Here's the drawing with two shaded views (mm, measured from the low corner). I have some questions. Give positions to 0.01 mm unless a question says otherwise; leave off trailing zeros. Loops run counter-clockwise (first coordinate to the right, second up) from the corner with the lowest first, then second, coordinate; pieces in that order, holes last. Notation, with made-up numbers: (-29, 23.25) -> (11, 23.25) arc R32 ccw to (11, 52.25) -> close; hole circle Ø6 at (40, 81). An arc over 180 degrees is marked (long way). Answer in a Markdown table with one row per item. Add a question column.
Item 1: If we section it at D-D (x = 72): Write out the boundary of the cut face in (y, z).
Item 2: For P1, Ø1.5, axis at y = 1, z = 13.5, coming from the +X side (1 decimal); P2, Ø3, axis at x = 73, y = 1.5, coming from the -Z side, each with a flat end and sliding along its axis, tell me the tip position at first contact or that it passes through.
Item 3: If we section it at C-C (z = 19): Write out the boundary of the cut face in (x, y), then the cut area to 3 significant figures.
Item 4: If we section it at B-B (z = 35.5): Write out the boundary of the cut face in (x, y) (1 decimal).
Item 5: If we section it at A-A (y = 3.3): Write out the boundary of the cut face in (x, z) (1 decimal).
Item 6: If I drill on line 1 (Z direction, x = 47.5, y = 4.45) (1 decimal); line 2 (Z direction, x = 44, y = 1); line 3 (Z direction, x = 52.5, y = 2.6), over which ranges is the centre line in solid material (lowest first)?
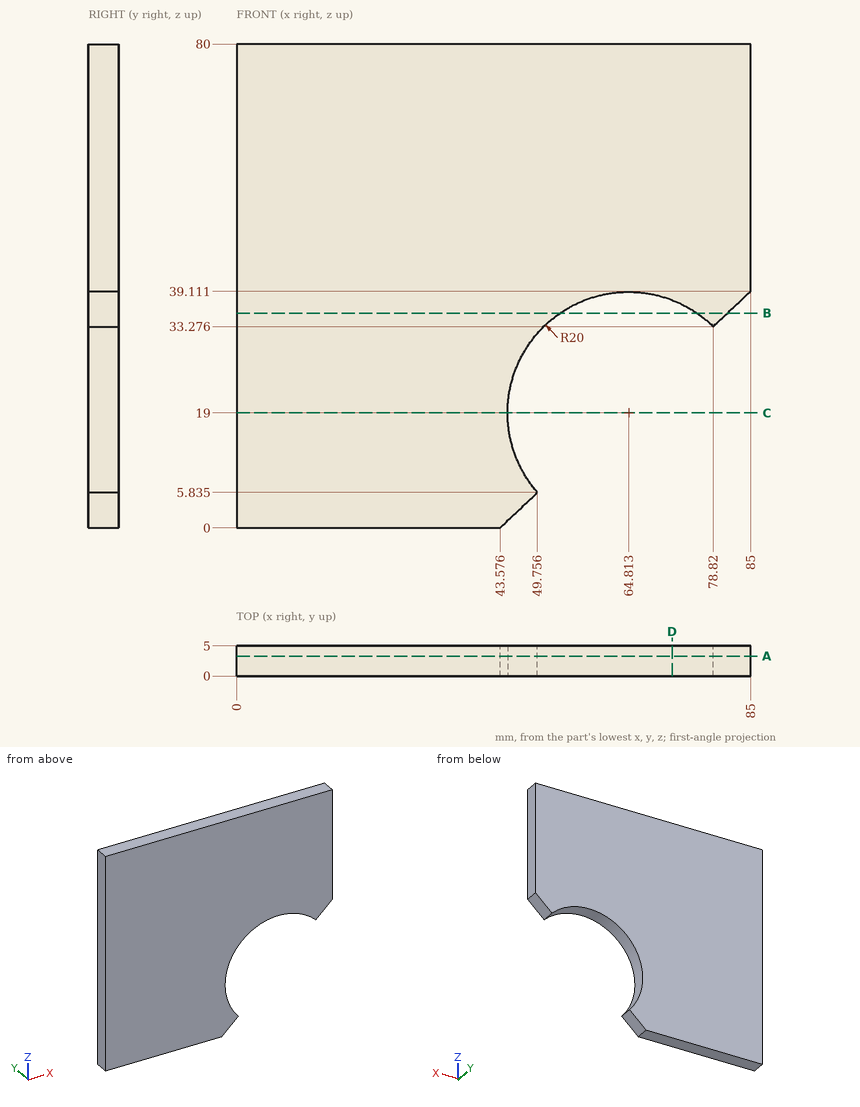
Recorded:
| question | item | result |
|---|---|---|
| 1 | outline | (0, 37.66) -> (5, 37.66) -> (5, 80) -> (0, 80) -> close |
| 2 | P1 | stops at x = 45.8 |
| 2 | P2 | stops at z = 36.5 |
| 3 | outline | (0, 0) -> (44.81, 0) -> (44.81, 5) -> (0, 5) -> close |
| 3 | area | 224 mm^2 |
| 4 | outline | (0, 0) -> (53.5, 0) -> (53.5, 5) -> (0, 5) -> close; (76.1, 0) -> (81.2, 0) -> (81.2, 5) -> (76.1, 5) -> close |
| 5 | outline | (0, 0) -> (43.6, 0) -> (49.8, 5.8) arc R20 cw to (78.8, 33.3) -> (85, 39.1) -> (85, 80) -> (0, 80) -> close |
| 6 | line 1 | z = 3.7 to 9, 29 to 80 |
| 6 | line 2 | z = 0.4 to 80 |
| 6 | line 3 | z = 34.76 to 80 |
